```python
from build123d import *

# Parameters (mm, degrees)
F0_R     = 15
F1_DEPTH = 40
F2_W     = 10
F2_H     = 5
F3_DEPTH = 20
F4_DEPTH = 15
F5_R     = 5
F6_DEPTH = 25
F7_R     = 152.5
F7_R_2   = 147.5
F8_DEPTH = 15
F9_DEPTH = 25


with BuildPart() as f1:
    # F0 (on Top) → F1 (new body)
    with BuildSketch(Plane.XY):
        Circle(F0_R)
        with BuildLine():
            ThreePointArc((9.5, 0), (8.2990963363, -4.6233105022), (5, -8.0777472107))
            ThreePointArc((5, -8.0777472107), (0, -9.5), (-5, -8.0777472107))
            ThreePointArc((-5, -8.0777472107), (-4.6233105022, 8.2990963363), (9.5, 0))
        make_face(mode=Mode.SUBTRACT)
        with BuildLine():
            ThreePointArc((-4.5, 0), (0, 4.5), (4.5, 0))
            Line((4.5, 0), (5, 0))
            Line((5, 0), (5, -8.0777472107))
            ThreePointArc((5, -8.0777472107), (8.2990963363, -4.6233105022), (9.5, 0))
            ThreePointArc((9.5, 0), (-4.6233105022, 8.2990963363), (-5, -8.0777472107))
            Line((-5, -8.0777472107), (-5, 0))
            Line((-5, 0), (-4.5, 0))
        make_face()
        with BuildLine():
            Line((5, 0), (4.5, 0))
            ThreePointArc((4.5, 0), (0, -4.5), (-4.5, 0))
            Line((-4.5, 0), (-5, 0))
            Line((-5, 0), (-5, -8.0777472107))
            ThreePointArc((-5, -8.0777472107), (0, -9.5), (5, -8.0777472107))
            Line((5, -8.0777472107), (5, 0))
        make_face()
    extrude(amount=F1_DEPTH)

    # F2 (on Front) → F3 (join, symmetric)
    with BuildSketch(Plane.XZ):
        with Locations((0, 37.5)):
            Rectangle(F2_W, F2_H)
    extrude(amount=F3_DEPTH, both=True)

    # F0 (on Top) → F4 (cut)
    with BuildSketch(Plane.XY):
        with BuildLine():
            ThreePointArc((-4.5, 0), (0, 4.5), (4.5, 0))
            Line((4.5, 0), (5, 0))
            Line((5, 0), (5, -8.0777472107))
            ThreePointArc((5, -8.0777472107), (8.2990963363, -4.6233105022), (9.5, 0))
            ThreePointArc((9.5, 0), (-4.6233105022, 8.2990963363), (-5, -8.0777472107))
            Line((-5, -8.0777472107), (-5, 0))
            Line((-5, 0), (-4.5, 0))
        make_face()
        with BuildLine():
            Line((5, 0), (4.5, 0))
            ThreePointArc((4.5, 0), (0, -4.5), (-4.5, 0))
            Line((-4.5, 0), (-5, 0))
            Line((-5, 0), (-5, -8.0777472107))
            ThreePointArc((-5, -8.0777472107), (0, -9.5), (5, -8.0777472107))
            Line((5, -8.0777472107), (5, 0))
        make_face()
    extrude(amount=F4_DEPTH, mode=Mode.SUBTRACT)

    # F5 (on Front) → F6 (cut)
    with BuildSketch(Plane.XZ):
        Circle(F5_R)
    extrude(amount=F6_DEPTH, mode=Mode.SUBTRACT)

    # F7 (on Top) → F8 (cut)
    with BuildSketch(Plane.XY):
        with Locations((0, 150)):
            Circle(F7_R)
        with Locations((0, 150)):
            Circle(F7_R_2, mode=Mode.SUBTRACT)
    extrude(amount=F8_DEPTH, mode=Mode.SUBTRACT)

    # F9 (cut): a face of the model
    f9_faces = [f1.faces().sort_by_distance(p)[0] for p in [
        (0, 0, 35),
    ]]
    extrude(f9_faces, amount=-F9_DEPTH, mode=Mode.SUBTRACT)


solid = f1.part
```
Could you check a few things on this model? Use its own coordinates, in mm. A direction names the side the tool comes from. Round coordinates to 2 decimals unless told otherwise and drop trailing zeros. Loops run counter-clockwise (first coordinate to the right, second up) from the corner with the lowest first, then second, coordinate; pieces in that order, holes last. Notation, with made-up numbers: (54.5, -26.75) - (67.5, -26.75) arc R8 cw to (67.5, -15.75) - close; hole circle Ø6 at (-23.75, -16). An arc over 180 degrees is marked (long way). Answer in a Markdown table with one row per item. Add a question column.
(1) I need wall thicknesses on line 1 along X through (y, z) = (0, 25.5); line 2 along Z through (x, y) = (7, -1.5). Which ranges of each line are inside material? Lowest first, please.
(2) I'm going to push flat-ended pins straight in: pin 1 (1.8 mm diameter, centred on x = -1, y = 16, fed in from -Z); pin 2 (8 mm diameter, centred on y = 10.5, z = 35, fed in from +X); pin 3 (6 mm diameter, centred on x = -10.5, z = 17, fed in from +Y). Where does each tip first touch, or does it pass through?
(3) If we mould it in two halves opening along Y, with no side actions, what happens to faces 5 (the face through (0, 20, 38)), 6 (the face through (-5, 17, 37)), 7 (the face through (4.292, -1.352, 27.325))? For each: pulls with the +Y half, pulls with the -Y half, needs draft (parallel to the pull), parting line crosses it, or undercut.
(4) If we section it at A-A (y = 0): Please give me the cut outline in (x, z).
(5) For faces 1 (the face through (0, -11, 5)), 2 (the face through (5, -17, 37)), 3 (the face through (-11.91, 2.98, 7.4)), 4 (the face through (-4, 4, 15)), which set-ups out of +Z, -Z, +X, -X, +Y, -Y let a thin tool reach every point of the face, with its end or its side?
(6) If we section it at B-B (x = 0): Please give me the cut outline in (y, z), plus the area to 4 significant figures.
(7) If we section it at D-D (z = 24.5): Please give me the cut outline in (x, y), plus the area to 3 significant figures.
(8) If we section it at C-C (x = -7.5): Please give me the cut outline in (y, z), plus the area to 3 significant figures.
Model answer:
| question | item | result |
|---|---|---|
| 1 | line 1 | x = -15 to -4.5, 4.5 to 15 |
| 1 | line 2 | z = 15 to 40 |
| 2 | pin 1 | stops at z = 35 |
| 2 | pin 2 | stops at x = 13.52 |
| 2 | pin 3 | stops at y = 12.99 |
| 3 | face 5 | pulls with the +Y half |
| 3 | face 6 | needs draft |
| 3 | face 7 | undercut |
| 4 | outline | (-15, 15) - (-4.5, 15) - (-4.5, 40) - (-15, 40) - close; (4.5, 15) - (15, 15) - (15, 40) - (4.5, 40) - close |
| 5 | face 1 | -Z, -Y |
| 5 | face 2 | +Z, -Z, +X, -Y |
| 5 | face 3 | -Z, -X |
| 5 | face 4 | -Z |
| 6 | outline | (-20, 35) - (-15, 35) - (-15, 5) - (-9.5, 5) - (-9.5, 15) - (-4.5, 15) - (-4.5, 40) - (-20, 40) - close; (4.5, 15) - (9.5, 15) - (9.5, 0) - (15, 0) - (15, 35) - (20, 35) - (20, 40) - (4.5, 40) - close |
| 6 | area | 712.5 mm² |
| 7 | outline | circle Ø30 at (0, 0); hole circle Ø9 at (0, 0) |
| 7 | area | 643 mm² |
| 8 | outline | (-12.99, 0) - (-5.83, 0) - (-5.83, 15) - (5.83, 15) - (5.83, 0) - (12.99, 0) - (12.99, 40) - (-12.99, 40) - close |
| 8 | area | 864 mm² |
